Verification items for the finished model (mm, model axes). Give positions to 0.01 mm unless a question says otherwise; leave off trailing zeros. Loops run counter-clockwise (first coordinate to the right, second up) from the corner with the lowest first, then second, coordinate; pieces in that order, holes last. Notation, with made-up numbers: (33, -20) - (67, -20) arc R34 ccw to (67, 13) - close; hole circle Ø11 at (-37.75, 15.25). An arc over 180 degrees is marked (long way). Put each result on its own line as item: value. Start each with the question number.
```python
from build123d import *

# Parameters (mm, degrees)
SKETCH1_W           = 50.8
SKETCH1_H           = 225.425
SKETCH1_R           = 15.875
SKETCH1_R_2         = 2.4892
BOSS_EXTRUDE1_DEPTH = 25.4
SKETCH2_R           = 2.4892
CUT_EXTRUDE1_DEPTH  = 233.469848851
SKETCH3_W           = 44.45
SKETCH3_H           = 19.05
CUT_EXTRUDE2_DEPTH  = 233.469848884
SKETCH4_W           = 50.8
SKETCH4_H           = 142.24
CUT_EXTRUDE3_DEPTH  = 233.469848851


with BuildPart() as part:
    # Sketch1 → Boss-Extrude1 (new body)
    with BuildSketch(Plane.XY):
        with Locations((25.4, 112.7125)):
            Rectangle(SKETCH1_W, SKETCH1_H)
        with Locations((25.4, 196.85)):
            Circle(SKETCH1_R, mode=Mode.SUBTRACT)
        with Locations((25.4, 9.525)):
            Circle(SKETCH1_R_2, mode=Mode.SUBTRACT)
        with Locations((38.1, 9.525)):
            Circle(SKETCH1_R_2, mode=Mode.SUBTRACT)
        with Locations((12.7, 9.525)):
            Circle(SKETCH1_R_2, mode=Mode.SUBTRACT)
        with Locations((12.7, 22.225)):
            Circle(SKETCH1_R_2, mode=Mode.SUBTRACT)
        with Locations((25.4, 22.225)):
            Circle(SKETCH1_R_2, mode=Mode.SUBTRACT)
        with Locations((38.1, 22.225)):
            Circle(SKETCH1_R_2, mode=Mode.SUBTRACT)
        with Locations((12.7, 34.925)):
            Circle(SKETCH1_R_2, mode=Mode.SUBTRACT)
        with Locations((25.4, 34.925)):
            Circle(SKETCH1_R_2, mode=Mode.SUBTRACT)
        with Locations((38.1, 34.925)):
            Circle(SKETCH1_R_2, mode=Mode.SUBTRACT)
        with Locations((12.7, 85.725)):
            Circle(SKETCH1_R_2, mode=Mode.SUBTRACT)
        with Locations((25.4, 85.725)):
            Circle(SKETCH1_R_2, mode=Mode.SUBTRACT)
        with Locations((38.1, 85.725)):
            Circle(SKETCH1_R_2, mode=Mode.SUBTRACT)
        with Locations((12.7, 98.425)):
            Circle(SKETCH1_R_2, mode=Mode.SUBTRACT)
        with Locations((25.4, 98.425)):
            Circle(SKETCH1_R_2, mode=Mode.SUBTRACT)
        with Locations((38.1, 98.425)):
            Circle(SKETCH1_R_2, mode=Mode.SUBTRACT)
        with Locations((12.7, 149.225)):
            Circle(SKETCH1_R_2, mode=Mode.SUBTRACT)
        with Locations((25.4, 149.225)):
            Circle(SKETCH1_R_2, mode=Mode.SUBTRACT)
        with Locations((38.1, 149.225)):
            Circle(SKETCH1_R_2, mode=Mode.SUBTRACT)
        with Locations((12.7, 161.925)):
            Circle(SKETCH1_R_2, mode=Mode.SUBTRACT)
        with Locations((25.4, 161.925)):
            Circle(SKETCH1_R_2, mode=Mode.SUBTRACT)
        with Locations((38.1, 161.925)):
            Circle(SKETCH1_R_2, mode=Mode.SUBTRACT)
    extrude(amount=BOSS_EXTRUDE1_DEPTH)

    # Sketch2 → Cut-Extrude1 (cut, through all)
    with BuildSketch(Plane(origin=(50.8, 0, 0), x_dir=(0, 0, -1), z_dir=(1, 0, 0))):
        with Locations((-12.7, 9.525)):
            Circle(SKETCH2_R)
        with Locations((-12.7, 22.225)):
            Circle(SKETCH2_R)
        with Locations((-12.7, 34.925)):
            Circle(SKETCH2_R)
        with Locations((-12.7, 47.625)):
            Circle(SKETCH2_R)
        with Locations((-12.7, 60.325)):
            Circle(SKETCH2_R)
        with Locations((-12.7, 73.025)):
            Circle(SKETCH2_R)
        with Locations((-12.7, 85.725)):
            Circle(SKETCH2_R)
        with Locations((-12.7, 98.425)):
            Circle(SKETCH2_R)
        with Locations((-12.7, 111.125)):
            Circle(SKETCH2_R)
        with Locations((-12.7, 123.825)):
            Circle(SKETCH2_R)
        with Locations((-12.7, 136.525)):
            Circle(SKETCH2_R)
        with Locations((-12.7, 149.225)):
            Circle(SKETCH2_R)
        with Locations((-12.7, 161.925)):
            Circle(SKETCH2_R)
        with Locations((-12.7, 174.625)):
            Circle(SKETCH2_R)
        with Locations((-12.7, 187.325)):
            Circle(SKETCH2_R)
        with Locations((-12.7, 200.025)):
            Circle(SKETCH2_R)
        with Locations((-12.7, 212.725)):
            Circle(SKETCH2_R)
    extrude(amount=-CUT_EXTRUDE1_DEPTH, mode=Mode.SUBTRACT)

    # Sketch3 → Cut-Extrude2 (cut, through all)
    with BuildSketch(Plane(origin=(0, 225.425, 0), x_dir=(1, 0, 0), z_dir=(0, 1, 0))):
        with Locations((25.4, -12.7)):
            Rectangle(SKETCH3_W, SKETCH3_H)
    extrude(amount=-CUT_EXTRUDE2_DEPTH, mode=Mode.SUBTRACT)

    # Sketch4 → Cut-Extrude3 (cut, through all)
    with BuildSketch(Plane.XY.offset(25.4)):
        with Locations((25.4, 71.12)):
            Rectangle(SKETCH4_W, SKETCH4_H)
    extrude(amount=-CUT_EXTRUDE3_DEPTH, mode=Mode.SUBTRACT)


solid = part.part
```
1) Scan lines: line 1 along Y through (x, z) = (25.4, 2.5) (3 decimals); line 2 along X through (y, z) = (183, 5) (3 decimals); line 3 along Z through (x, y) = (19, 167.5) (3 decimals). Record each from-to range of solid material in increasing order. Write a range as from..to.
2) Section check B-B, the plane z = 6. Enter the section's corners in (x, y) (3 decimals).
3) Section check A-A, the plane x = 25.4. State how many separate pieces and enclosed holes the cut face has, plus the area to 3 significant figures.
4) Draft check along X on faces 1 (the face through (1.61, 172.417, 11.551)), 2 (the face through (26.549, 159.717, 1.565)), 3 (the face through (12.16, 159.495, 1.565)). Enter one of: pulls with the +X half, pulls with the -X half, needs draft (parallel to the pull), parting line crosses it, or undercut.
5) Section check C-C, the plane y = 208.5. Enter the section's corners in (x, z) (3 decimals).
Results are:
1. line 1: y = 142.24..146.736, 151.714..159.436, 164.414..180.975, 212.725..225.425
1. line 2: x = 0..3.175, 47.625..50.8
1. line 3: z = 0..3.175, 22.225..25.4
2. outline: (0, 142.24) - (3.175, 142.24) - (3.175, 225.425) - (0, 225.425) - close; (47.625, 142.24) - (50.8, 142.24) - (50.8, 225.425) - (47.625, 225.425) - close
3. separate pieces: 8
3. enclosed holes: 0
3. area: 263 mm2
4. face 1: needs draft
4. face 2: undercut
4. face 3: undercut
5. outline: (0, 0) - (14.616, 0) - (14.616, 3.175) - (3.175, 3.175) - (3.175, 22.225) - (14.616, 22.225) - (14.616, 25.4) - (0, 25.4) - close; (36.184, 0) - (50.8, 0) - (50.8, 25.4) - (36.184, 25.4) - (36.184, 22.225) - (47.625, 22.225) - (47.625, 3.175) - (36.184, 3.175) - close
